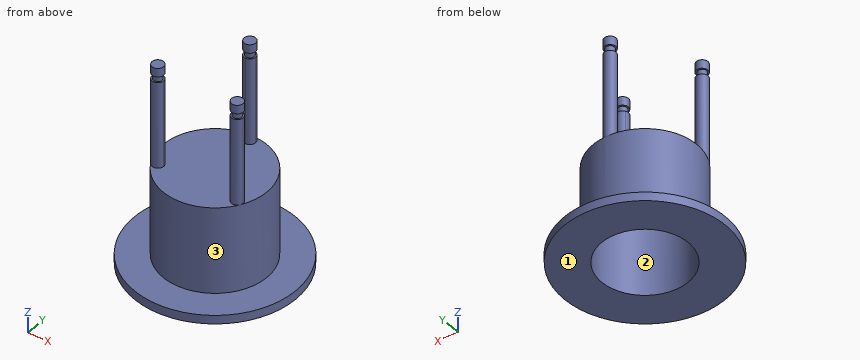
from build123d import *

# Parameters (mm, degrees)
F0_W      = 10
F0_H      = 3
F3_DEPTH  = 30
F4_R      = 1.5
F5_DEPTH  = 2
F6_R      = 2
F7_DEPTH  = 3
F8_R      = 1.5
F9_DEPTH  = 2
F10_R     = 2
F11_DEPTH = 3
F12_R     = 1.5
F13_DEPTH = 2
F14_R     = 2
F15_DEPTH = 3


with BuildPart() as f1:
    # F0 (on Front) → F1 (revolve)
    with BuildSketch(Plane.XZ):
        Polygon((18, -30), (18, -3), (15.029126, -3), (15.029126, -33), (18, -33), align=None)
        Polygon((15.029126, -3), (18, -3), (18, 0), (0, 0), (0, -3), align=None)
        with Locations((23, -31.5)):
            Rectangle(F0_W, F0_H)
    revolve(axis=Axis((0, 0, -1.5), (0, 0, 1)))

    # F2 (on face) → F3 (join)
    with BuildSketch(Plane.XY):
        with BuildLine():
            ThreePointArc((0, 14), (1.414214, 14.585786), (2, 16))
            ThreePointArc((2, 16), (-1.414214, 17.414214), (0, 14))
        make_face()
        with BuildLine():
            ThreePointArc((15.856406, -8), (14.374045, -6.068148), (12.124356, -7))
            ThreePointArc((12.124356, -7), (13.338768, -9.931852), (15.856406, -8))
        make_face()
        with BuildLine():
            ThreePointArc((-11.856406, -8), (-11.924555, -7.482362), (-12.124356, -7))
            ThreePointArc((-12.124356, -7), (-15.788258, -8.517638), (-11.856406, -8))
        make_face()
    extrude(amount=F3_DEPTH)

    # F4 (on face) → F5 (join)
    with BuildSketch(Plane.XY.offset(30)):
        with Locations((13.856406, -8)):
            Circle(F4_R)
    extrude(amount=F5_DEPTH)

    # F6 (on face) → F7 (join)
    with BuildSketch(Plane.XY.offset(32)):
        with Locations((13.856406, -8)):
            Circle(F6_R)
    extrude(amount=F7_DEPTH)

    # F8 (on face) → F9 (join)
    with BuildSketch(Plane.XY.offset(30)):
        with Locations((0, 16)):
            Circle(F8_R)
    extrude(amount=F9_DEPTH)

    # F10 (on face) → F11 (join)
    with BuildSketch(Plane.XY.offset(32)):
        with Locations((0, 16)):
            Circle(F10_R)
    extrude(amount=F11_DEPTH)

    # F12 (on face) → F13 (join)
    with BuildSketch(Plane.XY.offset(30)):
        with Locations((-13.856406, -8)):
            Circle(F12_R)
    extrude(amount=F13_DEPTH)

    # F14 (on face) → F15 (join)
    with BuildSketch(Plane.XY.offset(32)):
        with Locations((-13.856406, -8)):
            Circle(F14_R)
    extrude(amount=F15_DEPTH)


solid = f1.part
Work out the finished part from the listing and answer in its coordinate system (mm). Face numbers are marked on the shaded views. Give positions to 0.01 mm unless a question says otherwise; leave off trailing zeros. Loops run counter-clockwise (first coordinate to the right, second up) from the corner with the lowest first, then second, coordinate; pieces in that order, holes last. Notation, with made-up numbers: (62.25, 63) - (67.25, 63) arc R18 ccw to (67.25, 93) - close; hole circle Ø8 at (72, 31). An arc over 180 degrees is marked (long way). Answer in a Markdown table with one row per item.
(1) Flat-ended cylindrical pins translate along their axes: pin 1 Ø18 at (x, y) = (-4, 0) entering from +Z; pin 2 Ø5 at (x, y) = (-16.5, -5.5) entering from +Z; pin 3 Ø2 at (y, z) = (15, 14) entering from +X; pin 4 Ø10 at (x, z) = (-16.5, -7) entering from +Y. Find the tip coordinate at first contact, or state that the pin passes through.
Results list:
| item | result |
|---|---|
| pin 1 | stops at z = 0 |
| pin 2 | stops at z = 35 |
| pin 3 | stops at x = 2 |
| pin 4 | stops at y = 13.85 |
(2) Section B-B (z = 17) is taken. Give the vertices of the cut face in (x, y).
Results list:
| item | result |
|---|---|
| outline | (-12.12, -7) arc R2 ccw (long way) to (-11.86, -8) arc R2 ccw to start; (0, 14) arc R2 ccw to (2, 16) arc R2 ccw (long way) to start; (12.12, -7) arc R2 ccw (long way) to (15.86, -8) arc R2 ccw to start |
(3) Section C-C (z = -9) is taken. Give the vertices of the cut face in (x, y), and give its area (3 significant figures).
Results list:
| item | result |
|---|---|
| outline | circle Ø36 at (0, 0); hole circle Ø30.06 at (0, 0) |
| area | 308 mm² |
(4) For a pull along X with two mould halves and no side action, classify the marked faces 1, 2 and 3 as pulls with the +X half, pulls with the -X half, needs draft (parallel to the pull), parting line crosses it, or undercut.
Results list:
| item | result |
|---|---|
| face 1 | needs draft |
| face 2 | undercut |
| face 3 | parting line crosses it |
(5) Section D-D (x = 9.5) is taken. Give the vertices of the cut face in (y, z).
Results list:
| item | result |
|---|---|
| outline | (-26.34, -33) - (-11.65, -33) - (-11.65, -3) - (11.65, -3) - (11.65, -33) - (26.34, -33) - (26.34, -30) - (15.29, -30) - (15.29, 0) - (-15.29, 0) - (-15.29, -30) - (-26.34, -30) - close |
(6) Section A-A (y = 0) is taken. Give the vertices of the cut face in (x, z).
Results list:
| item | result |
|---|---|
| outline | (-28, -33) - (-15.03, -33) - (-15.03, -3) - (15.03, -3) - (15.03, -33) - (28, -33) - (28, -30) - (18, -30) - (18, 0) - (-18, 0) - (-18, -30) - (-28, -30) - close |
(7) Consider L1, parallel to Y at x = 0, z = -26.5; L2, parallel to Z at x = -8, y = -10; L3, parallel to X at y = -13.5, z = -14.5. Determine where each line is inside the solid, lowest interval first. Write a range as [from, to].
Results list:
| item | result |
|---|---|
| L1 | y = [-18, -15.03], [15.03, 18] |
| L2 | z = [-3, 0] |
| L3 | x = [-11.91, -6.6], [6.6, 11.91] |
